Work out the finished part from the listing and answer in its coordinate system (mm). Give positions to 0.01 mm unless a question says otherwise; leave off trailing zeros. Write each loop counter-clockwise with the first axis right and the second up, starting at its lowest first coordinate (ties: lowest second). Pieces come first, ordered by that corner, then holes. Notation, with made-up numbers: (-31, 38.5) -> (-15, 38.5) arc R37 cw to (-15, 77.5) -> close; hole circle Ø6 at (-6, 34). An arc over 180 degrees is marked (long way). Use a Markdown table: item, result. Add a question column.
Q1. Section B-B, the plane z = 14 is taken. Give the vertices of the cut face in (x, y).
Q2. Consider line 1 (Z direction, x = -4, y = 0); line 2 (Z direction, x = 0, y = -0.25); line 3 (Z direction, x = 0.25, y = 0). Determine where each line is inside the solid, lowest interval first.
Q3. Section A-A, the plane x = 3.5 is taken. Give the vertices of the cut face in (y, z), plus the area to 3 significant figures.
Q4. This flat-tipped pin is pushed along its axis until it touches: pin 1 Ø1.5 at (y, z) = (-1, 110) entering from +X. Where does it stop, or does it pass through?
Autodesk Inventor part; units mm, degrees
ref_plane "YZ Plane" through (0, 0, 0) normal (1, 0, 0) x (0, 1, 0)
ref_plane "XZ Plane" through (0, 0, 0) normal (0, 1, 0) x (-1, 0, 0)
ref_plane "XY Plane" through (0, 0, 0) normal (0, 0, 1) x (1, 0, 0)
sketch "Sketch1" plane through (0, 0, 0) normal (0, 0, 1) x (1, 0, 0)
  circle A0 centre (0, 0) radius 6.35
  dimension "d0" = 12.7
extrude "Extrusion1" add sketch "Sketch1" along normal blind 203.2
sketch "Sketch4" plane through (0, 0, 0) normal (0, 1, 0) x (-1, 0, 0)
  line L0 (0, 0) -> (0, 1.524)
  line L1 (6.35, 203.2) -> (-6.35, 203.2)
  line L2 (0, 203.2) -> (0, 201.676)
  circle A0 centre (0, 201.676) radius 1.27
  circle A1 centre (0, 1.524) radius 1.27
  dimension "d13" = 1.524
  dimension "d15" = 1.524
  dimension "d16" = 2.54
  dimension "d19" = 2.54
extrude "Extrusion4" cut sketch "Sketch4" along normal mid plane 15.24
sketch "Sketch5" plane through (0, 0, 0) normal (0, 1, 0) x (-1, 0, 0)
  line L0 (0, 1.524) -> (-1.27, 1.524)
  line L1 (-6.35, 0) -> (6.35, 0)
  line L2 (-1.27, 0) -> (1.27, 0)
  line L3 (1.27, 1.524) -> (0, 1.524)
  line L4 (1.27, 1.524) -> (6.35, 1.524)
  line L5 (6.35, 0) -> (6.35, 203.2)
  line L6 (6.35, 1.524) -> (-6.35, 1.524)
  line L7 (-6.35, 1.524) -> (-6.35, 0)
  line L8 (-6.35, 0) -> (6.35, 0)
  line L9 (6.35, 0) -> (6.35, 1.524)
  line L10 (6.35, 203.2) -> (-6.35, 203.2)
  line L11 (-6.35, 203.2) -> (6.35, 203.2)
  line L12 (6.35, 203.2) -> (6.35, 201.676)
  line L13 (6.35, 201.676) -> (-6.35, 201.676)
  line L14 (-6.35, 201.676) -> (-6.35, 203.2)
  point P0 (0, 0)
  dimension "d20" = 1.524
  dimension "d21" = 1.27
  dimension "d26" = 12.7
  dimension "d27" = 1.524
sketch "Sketch7" plane through (0, 0, 0) normal (1, 0, 0) x (0, 1, 0)
  line L0 (0, 0) -> (0, 50.8)
  circle A0 centre (0, 50.8) radius 1.27
  line L1 (0, 50.8) -> (0, 101.6)
  circle A1 centre (0, 101.6) radius 1.27
  line L2 (0, 101.6) -> (0, 152.4)
  circle A2 centre (0, 152.4) radius 1.27
  dimension "d42" = 50.8
  dimension "d43" = 2.54
  dimension "d44" = 50.8
  dimension "d45" = 2.54
  dimension "d46" = 50.8
  dimension "d47" = 2.54
extrude "Extrusion8" cut sketch "Sketch7" along normal mid plane 25.4
extrude "Extrusion9" cut sketch "Sketch5" along normal mid plane 25.4 contours L13 L14 L10 L5
properties part number "Straw"
Result set:
| question | item | result |
|---|---|---|
| 1 | outline | circle Ø12.7 at (0, 0) |
| 2 | line 1 | z = 0 to 49.53, 52.07 to 100.33, 102.87 to 151.13, 153.67 to 201.68 |
| 2 | line 2 | z = 0 to 0.25, 2.79 to 49.55, 52.05 to 100.35, 102.85 to 151.15, 153.65 to 200.41 |
| 2 | line 3 | z = 0 to 0.28, 2.77 to 49.53, 52.07 to 100.33, 102.87 to 151.13, 153.67 to 200.43 |
| 3 | outline | (-5.3, 0) -> (5.3, 0) -> (5.3, 201.68) -> (-5.3, 201.68) -> close; hole circle Ø2.54 at (0, 50.8); hole circle Ø2.54 at (0, 101.6); hole circle Ø2.54 at (0, 152.4) |
| 3 | area | 2,120 mm2 |
| 4 | pin 1 | stops at x = 6.35 |
